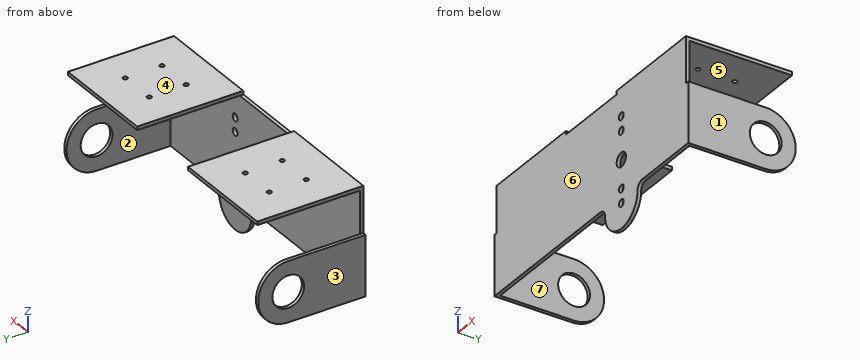
Autodesk Inventor part; units mm, degrees
ref_plane "Work Plane1" through (133.35, 0, 0) normal (1, 0, 0) x (0, 0, -1)
ref_plane "YZ Plane" through (0, 0, 0) normal (1, 0, 0) x (0, 1, 0)
ref_plane "XZ Plane" through (0, 0, 0) normal (0, 1, 0) x (-1, 0, 0)
sketch "Sketch1" plane through (0, 0, 0) normal (1, 0, 0) x (0, 1, 0)
  circle A0 centre (0, 0) radius 14.2875
  line L0 (-66.3768, 26.9875) -> (-66.3768, -26.9875)
  circle A1 centre (0, 0) radius 26.9875
  line L1 (0, 26.9875) -> (-66.3768, 26.9875)
  line L2 (0, -26.9875) -> (-66.3768, -26.9875)
  point P0 (-66.3768, 0)
  dimension "d0" = 28.575
  dimension "d1" = 66.3768
  dimension "d2" = 53.975
  dimension "d3" = 12.7
extrude "Extrusion1" add sketch "Sketch1" along normal blind 3.175
sketch "Sketch2" plane through (0, -66.3768, -26.9875) normal (0, -1, 0) x (1, 0, 0)
  line L0 (0, 0) -> (0, 53.975)
  line L1 (0, 53.975) -> (133.35, 53.975)
  line L2 (133.35, 53.975) -> (133.35, 0)
  line L3 (133.35, 0) -> (0, 0)
  line L4 (0, 0) -> (0, 53.975)
  point P0 (0, 26.9875)
  dimension "d6" = 53.975
  dimension "d7" = 133.35
extrude "Extrusion2" add sketch "Sketch2" along normal blind 3.175
mirror "Mirror1" about plane through (133.35, -66.3768, -26.9875) normal (1, 0, 0)
sketch "Sketch3" plane through (0, -66.3768, -26.9875) normal (0, 1, 0) x (1, 0, 0)
  line L0 (3.175, -53.975) -> (3.175, 0)
  line L1 (3.175, -53.975) -> (263.525, -53.975)
  line L2 (263.525, -53.975) -> (263.525, 0)
  line L3 (263.525, 0) -> (3.175, 0)
  circle A0 centre (174.625, -31.745) radius 6.35
  circle A1 centre (174.625, -6.345) radius 3.3528
  circle A2 centre (174.625, 6.355) radius 3.3528
  circle A3 centre (174.625, -57.145) radius 3.3528
  circle A4 centre (174.625, -69.845) radius 3.3528
  arc A5 (152.2222, -69.845) -> (197.0278, -69.845) centre (174.625, -69.845) ccw
  arc A6 (197.0278, 6.355) -> (152.2222, 6.355) centre (174.625, 6.355) ccw
  line L4 (263.525, 0) -> (3.175, 0)
  line L5 (3.175, -53.975) -> (263.525, -53.975)
  arc A7 (197.0278, 6.355) -> (203.3828, 0) centre (203.3828, 6.355) ccw
  arc A8 (145.8672, 0) -> (152.2222, 6.355) centre (145.8672, 6.355) ccw
  arc A9 (152.2222, -69.845) -> (136.3522, -53.975) centre (136.3522, -69.845) ccw
  arc A10 (212.8978, -53.975) -> (197.0278, -69.845) centre (212.8978, -69.845) ccw
  point P0 (0, -26.9875)
  dimension "d10" = 22.23
  dimension "d11" = 12.7
  dimension "d12" = 47.63
  dimension "d13" = 6.7056
  dimension "d14" = 6.7056
  dimension "d15" = 60.33
  dimension "d16" = 6.7056
  dimension "d17" = 3.17
  dimension "d18" = 6.7056
  dimension "d19" = 15.87
  dimension "d20" = 88.9
  dimension "d21" = 19.05
  dimension "d22" = 19.05
extrude "Extrusion3" add sketch "Sketch3" against normal blind 3.175 contours L0 L3 L2 L1 A3 | L1 A3 A10 A5 A9 | A8 A6 A7 L3 | A3 L1 | L1 A3 | A0 | A1 | A2 | A4
extrude "Extrusion4" cut sketch "Sketch3" against normal blind 3.175 contours A3 L1 | L1 A3 | A0 | A1 | A2 | A4
sketch "Sketch4" plane through (0, -66.3768, -26.9875) normal (0, 1, 0) x (1, 0, 0)
  line L0 (3.175, -53.975) -> (3.175, 0)
  line L1 (3.175, -53.975) -> (263.525, -53.975)
  line L2 (263.525, -53.975) -> (263.525, -92.2478)
  line L3 (263.525, -92.2478) -> (3.175, -92.2478)
  line L4 (3.175, -92.2478) -> (3.175, -53.975)
  arc A0 (152.2222, -69.845) -> (197.0278, -69.845) centre (174.625, -69.845) ccw
  line L5 (263.525, -53.975) -> (263.525, 0)
  arc A1 (152.2222, -69.845) -> (197.0278, -69.845) centre (174.625, -69.845) ccw
  circle A2 centre (174.625, -69.845) radius 3.3528
  circle A3 centre (174.625, -57.145) radius 3.3528
  arc A4 (173.533, -53.975) -> (175.717, -53.975) centre (174.625, -57.145) ccw
  point P0 (0, -26.9875)
  point P1 (174.625, -92.2478)
extrude "Extrusion5" add sketch "Sketch4" against normal blind 3.175 contours L1 A3 L2 L3 L4
sketch "Sketch5" plane through (3.175, -66.3768, 65.2603) normal (0, 0, 1) x (1, 0, 0)
  line L0 (0, -3.175) -> (0, 0)
  line L1 (0, -3.175) -> (95.25, -3.175)
  line L2 (95.25, -3.175) -> (95.25, 92.075)
  line L3 (95.25, 92.075) -> (0, 92.075)
  line L4 (0, 92.075) -> (0, -3.175)
  circle A0 centre (31.0727, 61.0023) radius 2.032
  circle A1 centre (64.1773, 61.0023) radius 2.032
  circle A2 centre (64.1773, 27.8977) radius 2.032
  circle A3 centre (31.0727, 27.8977) radius 2.032
  line L5 (29.0407, 61.0023) -> (0, 61.0023)
  line L6 (33.1047, 61.0023) -> (62.1453, 61.0023)
  line L7 (66.2093, 61.0023) -> (95.25, 61.0023)
  line L8 (31.0727, 63.0343) -> (31.0727, 92.075)
  line L9 (31.0727, 58.9703) -> (31.0727, 29.9297)
  line L10 (31.0727, 25.8657) -> (31.0727, -3.175)
  point P0 (-3.175, 66.3768)
  dimension "d29" = 95.25
  dimension "d30" = 95.25
  dimension "d31" = 4.064
  dimension "d32" = 4.064
  dimension "d33" = 4.064
  dimension "d34" = 4.064
extrude "Extrusion6" add sketch "Sketch5" along normal blind 3.175 contours L0 L4 L5 A0 L9 A3 L10 L1 | L10 A3 L9 A0 L6 A1 L7 L2 L1 | L4 L3 L8 A0 L5 | L7 A1 L6 A0 L8 L3 L2
ref_plane "Work Plane1" through (133.35, 0, 0) normal (1, 0, 0) x (0, 0, -1)
mirror "Mirror2" about plane through (133.35, 0, 0) normal (1, 0, 0) of "Extrusion6"
properties part number "Another Motor Bracket"
The model under review builds one solid part; all positions refer to its coordinate system, in mm. Face numbers are marked on the shaded views. A direction names the side the tool comes from. Coordinates: 2 decimals unless noted, no trailing zeros. Write each loop counter-clockwise with the first axis right and the second up, starting at its lowest first coordinate (ties: lowest second). Pieces come first, ordered by that corner, then holes. Notation, with made-up numbers: M 59,-26.75 L 74,-26.75 A33 ccw 74,9.25 Z; hole C -37,57 d4. An arc over 180 degrees is marked long. Put each result on its own line as item: value.
1) Clearance check with flat-ended pins moving along their axes: pin 1 Ø10 at (x, z) = (126.5, -28.5) entering from +Y; pin 2 Ø1 at (x, y) = (55, 0.5) entering from -Z; pin 3 Ø3.5 at (y, z) = (-8, 66.5) entering from +X (3 decimals). State where each tip first meets the part, or that it passes through.
Computed:
pin 1: stops at y = -66.38
pin 2: stops at z = 65.26
pin 3: stops at x = 263.525
2) Add section A-A on y = -60.5. Give the boundary of the cut face in (x, z) (1 decimal), then the cut area to 3 significant figures.
Computed:
outline: M 0,-27 L 3.2,-27 L 3.2,27 L 0,27 Z; M 3.2,65.3 L 98.4,65.3 L 98.4,68.4 L 3.2,68.4 Z; M 168.3,65.3 L 263.5,65.3 L 263.5,68.4 L 168.3,68.4 Z; M 263.5,-27 L 266.7,-27 L 266.7,27 L 263.5,27 Z
area: 948 mm2
3) Draft analysis for pull direction X (two halves, no side actions). For the marked faces 1, 2, 3 and 4, state which applies: released by +X, released by -X, zero draft, split by the parting line, or undercut.
Computed:
face 1: released by +X
face 2: undercut
face 3: released by -X
face 4: zero draft
4) Add section B-B on x = 135.5. Give the boundary of the cut face in (y, z).
Computed:
outline: M -69.55,-26.99 L -66.38,-26.99 L -66.38,65.26 L -69.55,65.26 Z
5) Wall thickness on probe 1 along X at (y, z) = (-20.5, 4) (3 decimals); probe 2 along Z at (x, y) = (203.5, 14); probe 3 along Y at (x, z) = (107, 29.5): over which ranges is each line inside the solid? List them lowest first. Write a range as [from, to].
Computed:
probe 1: x = [0, 3.175], [263.525, 266.7]
probe 2: z = [65.26, 68.44]
probe 3: y = [-69.55, -66.38]
6) Add section C-C on z = -42. Give the boundary of the cut face in (x, y), then the cut area to 3 significant figures.
Computed:
outline: M 153.96,-69.55 L 195.29,-69.55 L 195.29,-66.38 L 153.96,-66.38 Z
area: 131 mm2
7) For the marked faces 5, 6 and 7, list the 3-axis set-ups (+Z, -Z, +X, -X, +Y, -Y) from which the entire face can be reached by the end or side of a thin tool; tool diameter is ignored.
Computed:
face 5: -Z, +X, -X, +Y
face 6: +Z, -Z, +X, -X, -Y
face 7: -Z, +Y
